```python
from build123d import *

# Parameters (mm, degrees)
BOSS_EXTRUDE1_DEPTH = 80


with BuildPart() as part:
    # Sketch1 → Boss-Extrude1 (new body)
    with BuildSketch(Plane(origin=(0, 0, 0), x_dir=(1, 0, 0), z_dir=(0, 1, 0))):
        with BuildLine():
            Line((-1.75, 2.6), (-1.75, 4.415880433))
            ThreePointArc((-1.75, 4.415880433), (-4.75, 0), (-1.75, -4.415880433))
            Line((-1.75, -4.415880433), (-1.75, -2.6))
            Line((-1.75, -2.6), (1.75, -2.6))
            Line((1.75, -2.6), (1.75, -4.415880433))
            ThreePointArc((1.75, -4.415880433), (3.929058411, -2.669269563), (4.75, 0))
            ThreePointArc((4.75, 0), (3.929058411, 2.669269563), (1.75, 4.415880433))
            Line((1.75, 4.415880433), (1.75, 2.6))
            Line((1.75, 2.6), (-1.75, 2.6))
        make_face()
    extrude(amount=BOSS_EXTRUDE1_DEPTH)


solid = part.part
```
Design review of the part built by this model. Coordinates are the model's own, in mm. A direction names the side the tool comes from. Coordinates: 2 decimals unless noted, no trailing zeros. Loops run counter-clockwise (first coordinate to the right, second up) from the corner with the lowest first, then second, coordinate; pieces in that order, holes last. Notation, with made-up numbers: (0.5, 12.25) -> (22.5, 12.25) arc R14 ccw to (22.5, 24.25) -> close; hole circle Ø2 at (67.5, 23.25). An arc over 180 degrees is marked (long way). Answer as a JSON object with one key per item and string values.
Q1. Take a section at A-A on z = 3.5. Give the boundary of the cut face in (x, y).
Answer block:
{"outline": "(-3.21, 0) -> (-1.75, 0) -> (-1.75, 80) -> (-3.21, 80) -> close; (1.75, 0) -> (3.21, 0) -> (3.21, 80) -> (1.75, 80) -> close"}
Q2. Tool access review of faces 4 (the flat face through (1.75, 39, 3)), 5 (the flat face through (1.75, 39, -4)), 6 (the flat face through (0, 80, 0)): name each direction out of +Z, -Z, +X, -X, +Y, -Y from which nothing blocks a thin tool from reaching the whole face with its end or side.
Answer block:
{"face 4": "+Z, +Y, -Y", "face 5": "-Z, +Y, -Y", "face 6": "+Z, -Z, +X, -X, +Y"}
Q3. Take a section at D-D on z = -3.75. Give the boundary of the cut face in (x, y).
Answer block:
{"outline": "(-2.92, 0) -> (-1.75, 0) -> (-1.75, 80) -> (-2.92, 80) -> close; (1.75, 0) -> (2.92, 0) -> (2.92, 80) -> (1.75, 80) -> close"}
Q4. The part is to be moulded in two halves that separate along X. For faces 1 (the cylindrical face through (-4.75, 39.44, -0.08)), 2 (the flat face through (0, 39, 2.6)), 3 (the flat face through (0, 0, 0)), say which applies: +X half, -X half, draft (parallel to the pull), parting line (faces both ways), or undercut.
Answer block:
{"face 1": "-X half", "face 2": "undercut", "face 3": "draft"}
Q5. Clearance check with flat-ended pins moving along their axes: pin 1 Ø2 at (y, z) = (43, -3.5) entering from +X; pin 2 Ø3 at (y, z) = (71, -2.5) entering from -X; pin 3 Ø2 at (y, z) = (22.5, 3) entering from -X. State where each tip first meets the part, or that it passes through.
Answer block:
{"pin 1": "stops at x = 4.04", "pin 2": "stops at x = -4.64", "pin 3": "stops at x = -4.31"}
Q6. Take a section at C-C on x = 0.5. Give the boundary of the cut face in (y, z).
Answer block:
{"outline": "(0, -2.6) -> (80, -2.6) -> (80, 2.6) -> (0, 2.6) -> close"}
Q7. To check wall thickness, follow L1, parallel to Z at x = 1, y = 37.5; L2, parallel to X at y = 71, z = 2.75; L3, parallel to X at y = 32, z = 3.25. State the ranges of each line that lie inside material, in increasing order.
Answer block:
{"L1": "z = -2.6 to 2.6", "L2": "x = -3.87 to -1.75, 1.75 to 3.87", "L3": "x = -3.46 to -1.75, 1.75 to 3.46"}
Q8. Take a section at B-B on y = 39. Give the boundary of the cut face in (x, z), plus the area to 3 significant figures.
Answer block:
{"outline": "(-1.75, -4.42) -> (-1.75, -2.6) -> (1.75, -2.6) -> (1.75, -4.42) arc R4.75 ccw to (1.75, 4.42) -> (1.75, 2.6) -> (-1.75, 2.6) -> (-1.75, 4.42) arc R4.75 ccw to start", "area": "56.6 mm^2"}
